```python
from build123d import *
from OCP.BRepFilletAPI import BRepFilletAPI_MakeChamfer

# Parameters (mm, degrees)
SKETCH1_W           = 20
SKETCH1_H           = 20
BOSS_EXTRUDE1_DEPTH = 25
CIRPATTERN1_COUNT   = 5
CIRPATTERN1_ANGLE   = 160
CHAMFER1_SIZE       = 15
CHAMFER1_SIZE2      = 8.660254038


with BuildPart() as part:
    # Sketch1 → Boss-Extrude1 (new body)
    with BuildSketch(Plane.XY):
        with BuildLine():
            Line((-119, 0), (0, 0))
            ThreePointArc((0, 0), (-59.5, -59.5), (-119, 0))
        make_face()
        with Locations((-40, -25)):
            Rectangle(SKETCH1_W, SKETCH1_H, mode=Mode.SUBTRACT)
        with Locations((-79, -25)):
            Rectangle(SKETCH1_W, SKETCH1_H, mode=Mode.SUBTRACT)
    extrude(amount=BOSS_EXTRUDE1_DEPTH)

    # Sketch4 → Ø4.0mm Dowel Hole2 (revolve, cut)
    with BuildSketch(Plane(origin=(-0.903938696, -10.332066571, 12.5), x_dir=(0.1736481776669305, 0.9848077530122081, 0), z_dir=(0, 0, 1))):
        Polygon((0, 0), (0, 11.201721238), (2, 10), (2, 0.025), (2.025, 0), align=None)
    f_4_0mm_dowel_hole2 = revolve(axis=Axis((5.349590536, -11.434732499, 12.5), (-0.9848077530122081, 0.1736481776669305, 0)), mode=Mode.SUBTRACT)

    # CirPattern1: Ø4.0mm Dowel Hole2 ×5 about axis
    cirpattern1_axis = Axis((-59.5, 0, 0), (0, 0, -1))
    for i in range(1, CIRPATTERN1_COUNT):
        add(f_4_0mm_dowel_hole2.rotate(cirpattern1_axis, i * CIRPATTERN1_ANGLE / (CIRPATTERN1_COUNT - 1)), mode=Mode.SUBTRACT)

    # Chamfer1: one chamfer whose edges measure the first distance from different faces: ONE call of the kernel's chamfer builder (chamfer() names one face for all edges)
    chamfer1_edges_1 = [part.edges().sort_by_distance(p)[0] for p in [
        (-40, -15, 25),
    ]]
    chamfer1_side_1 = [part.faces().sort_by_distance(p)[0] for p in [
        (-40, -15, 12.5),
    ]]
    chamfer1_edges_2 = [part.edges().sort_by_distance(p)[0] for p in [
        (-79, -15, 25),
    ]]
    chamfer1_side_2 = [part.faces().sort_by_distance(p)[0] for p in [
        (-79, -15, 12.5),
    ]]
    chamfer1 = BRepFilletAPI_MakeChamfer(part.part.solid().wrapped)
    for e in chamfer1_edges_1:
        chamfer1.Add(CHAMFER1_SIZE, CHAMFER1_SIZE2, e.wrapped, chamfer1_side_1[0].wrapped)  # the first distance lies on this face
    for e in chamfer1_edges_2:
        chamfer1.Add(CHAMFER1_SIZE, CHAMFER1_SIZE2, e.wrapped, chamfer1_side_2[0].wrapped)  # the first distance lies on this face
    add(Compound.cast(chamfer1.Shape()), mode=Mode.REPLACE)


solid = part.part
```
The model under review builds one solid part; all positions refer to its coordinate system, in mm. A direction names the side the tool comes from. Round coordinates to 2 decimals unless told otherwise and drop trailing zeros. Write each loop counter-clockwise with the first axis right and the second up, starting at its lowest first coordinate (ties: lowest second). Pieces come first, ordered by that corner, then holes. Notation, with made-up numbers: (83, -30) - (91, -30) arc R27 cw to (91, -12) - close; hole circle Ø8 at (41, -33.75). An arc over 180 degrees is marked (long way). Answer as CSV lines item,"result". Start each with the question number.
(1) We need section B-B on y = -27.5. State the section outline as (x, z) points, plus the area to 3 significant figures.
(2) We need section A-A on z = 6.25. State the section outline as (x, y) points, plus the area to 3 significant figures.
(3) Draft analysis for pull direction Z (two halves, no side actions). For faces 1 (the flat face through (-59, -23, 0)), 2 (the flat face through (-59, -29, 25)), 3 (the cylindrical face through (-93.11, -43.02, 11.9)), state which applies: pulls with the +Z half, pulls with the -Z half, needs draft (parallel to the pull), parting line crosses it, or undercut.
(4) We need section C-C on x = -47.5. State the section outline as (y, z) points.
(5) To check wall thickness, follow line 1 (X direction, y = -31.5, z = 9); line 2 (Z direction, x = -59.5, y = -54.25); line 3 (X direction, y = -10, z = 23.75). State the ranges of each line that lie inside material, in increasing order.
(6) We need section D-D on y = -52.5. State the section outline as (x, z) points, plus the area to 3 significant figures.
(7) For faces 4 (the flat face through (-40.14, -10.61, 17.6)), 5 (the flat face through (-79, -15, 5)), 6 (the conical face through (-59.34, -48.51, 12.81)), 7 (the conical face through (-107.21, -8.75, 12.4)), list the 3-axis set-ups (+Z, -Z, +X, -X, +Y, -Y) from which the entire face can be reached by the end or side of a thin tool; tool diameter is ignored.
(8) For pin 1 Ø12 at (y, z) = (-7.5, 20.5) entering from -X; pin 2 Ø8 at (x, z) = (-75.5, 6) entering from -Y; pin 3 Ø5 at (x, z) = (-75.5, 21.5) entering from -Y, all flat-tipped, find the tip position at first contact; note any pin that passes through.
Worked answers:
1,outline,"(-112.26, 0) - (-89, 0) - (-89, 25) - (-112.26, 25) - close; (-69, 0) - (-50, 0) - (-50, 25) - (-69, 25) - close; (-30, 0) - (-6.74, 0) - (-6.74, 25) - (-30, 25) - close"
1,area,"1,640 mm²"
2,outline,"(-119, 0) arc R59.5 ccw to (0, 0) - close; hole (-89, -35) - (-69, -35) - (-69, -15) - (-89, -15) - close; hole (-50, -35) - (-30, -35) - (-30, -15) - (-50, -15) - close"
2,area,"4,760 mm²"
3,face 1,"pulls with the -Z half"
3,face 2,"pulls with the +Z half"
3,face 3,"undercut"
4,outline,"(-58.28, 0) - (-35, 0) - (-35, 25) - (-58.28, 25) - close; (-15, 0) - (0, 0) - (0, 25) - (-6.34, 25) - (-15, 10) - close"
5,line 1,"-109.98 to -89, -69 to -50, -30 to -9.02"
5,line 2,"0 to 10.5, 14.5 to 25"
5,line 3,"-118.15 to -89, -69 to -50, -30 to -0.85"
6,outline,"(-87.5, 0) - (-31.5, 0) - (-31.5, 25) - (-87.5, 25) - close; hole circle Ø4 at (-59.5, 12.5)"
6,area,"1,390 mm²"
7,face 4,"+Z"
7,face 5,"+Z, -Z"
7,face 6,"-Y"
7,face 7,"none"
8,pin 1,"x = -118.98"
8,pin 2,"y = -58.28"
8,pin 3,"y = -57.95"
